Autodesk Fusion 360 part; units mm, degrees
sketch "Sketch1" plane through (0, 0, 0) normal (0, 1, 0) x (1, 0, 0)
  line L0 (0, 0) -> (7, 0)
  line L1 (7, 0) -> (7, -4)
  line L2 (7, -4) -> (10, -4)
  line L3 (0, -10) -> (0, 0)
  line L4 (0, -10) -> (2, -10)
  arc A0 (2, -10) -> (10, -4) centre (2, -1.6667) ccw
  dimension "d1" = 7
  dimension "d2" = 4
  dimension "d3" = 3
  dimension "d4" = 2
  dimension "d5" = 10
revolve "Revolve1" add sketch "Sketch1" angle 360 about axis through (0, 0, 10) along (0, 0, -1)
sketch "Sketch2" plane through (0, 0, 0) normal (0, 0, -1) x (1, 0, 0)
  circle A0 centre (0, 0) radius 7
  line L0 (1.55, 1.05) -> (1.55, -1.05)
  line L1 (-1.55, 1.05) -> (-1.55, -1.05)
  line L2 (0.55, -2.05) -> (-0.55, -2.05)
  line L3 (0.55, 2.05) -> (-0.55, 2.05)
  arc A1 (0.55, -2.05) -> (1.55, -1.05) centre (0.55, -1.05) ccw
  arc A2 (-0.55, 2.05) -> (-1.55, 1.05) centre (-0.55, 1.05) ccw
  arc A3 (-1.55, -1.05) -> (-0.55, -2.05) centre (-0.55, -1.05) ccw
  arc A4 (1.55, 1.05) -> (0.55, 2.05) centre (0.55, 1.05) ccw
  point P0 (0, -2.05)
  point P1 (1.55, 2.05)
  point P2 (1.55, -2.05)
  point P3 (1.55, 0)
  point P4 (-1.55, 2.05)
  dimension "d11" = 4.1
  dimension "d12" = 3.1
  dimension "d13" = 1
extrude "Extrude1" cut sketch "Sketch2" against normal blind 2.5 contours L0 L1 L2 L3 A1 A2 A3 A4
The model under review builds one solid part; all positions refer to its coordinate system, in mm. A direction names the side the tool comes from. Round coordinates to 2 decimals unless told otherwise and drop trailing zeros. Loops run counter-clockwise (first coordinate to the right, second up) from the corner with the lowest first, then second, coordinate; pieces in that order, holes last.
1) Wall thickness on line 1 along Z through (x, y) = (-0.5, -6.75); line 2 along X through (y, z) = (-6.5, 6); line 3 along Z through (x, y) = (7, -4.5): over which ranges is each line inside the solid? List them lowest first.
Values follow:
line 1: z = 0 to 8.5
line 2: x = -6.39 to 6.39
line 3: z = 4 to 7.1
2) Tool access review of faces 4 (the face through (-1.265, 1.749, 1.232)), 5 (the face through (-2, 0, 0)): name each direction out of +Z, -Z, +X, -X, +Y, -Y from which nothing blocks a thin tool from reaching the whole face with its end or side.
Values follow:
face 4: -Z
face 5: -Z, +X, -X, +Y, -Y
3) Clearance check with flat-ended pins moving along their axes: P1, Ø2.5, axis at y = -0.5, z = 2, coming from the +X side; P2, Ø0.6, axis at x = 0.5, z = 1.5, coming from the -Y side; P3, Ø4, axis at y = 2, z = 3, coming from the +X side. State where each tip first meets the part, or that it passes through.
Values follow:
P1: stops at x = 7
P2: stops at y = -7
P3: stops at x = 10
4) The part is to be moulded in two halves that separate along X. For faces 1 (the face through (0, 0, 10)), 2 (the face through (-1.55, 0, 1)), 3 (the face through (6.466, -2.681, 2.028)), say which applies: pulls with the +X half, pulls with the -X half, needs draft (parallel to the pull), parting line crosses it, or undercut.
Values follow:
face 1: needs draft
face 2: undercut
face 3: parting line crosses it
5) Consider section A-A on z = 0.5. State the section outline as (x, y) points, then the cut area to 3 significant figures.
Values follow:
outline: circle Ø14 at (0, 0); hole (-1.55, -1.05) arc R1 ccw to (-0.55, -2.05) - (0.55, -2.05) arc R1 ccw to (1.55, -1.05) - (1.55, 1.05) arc R1 ccw to (0.55, 2.05) - (-0.55, 2.05) arc R1 ccw to (-1.55, 1.05) - close
area: 142 mm2
